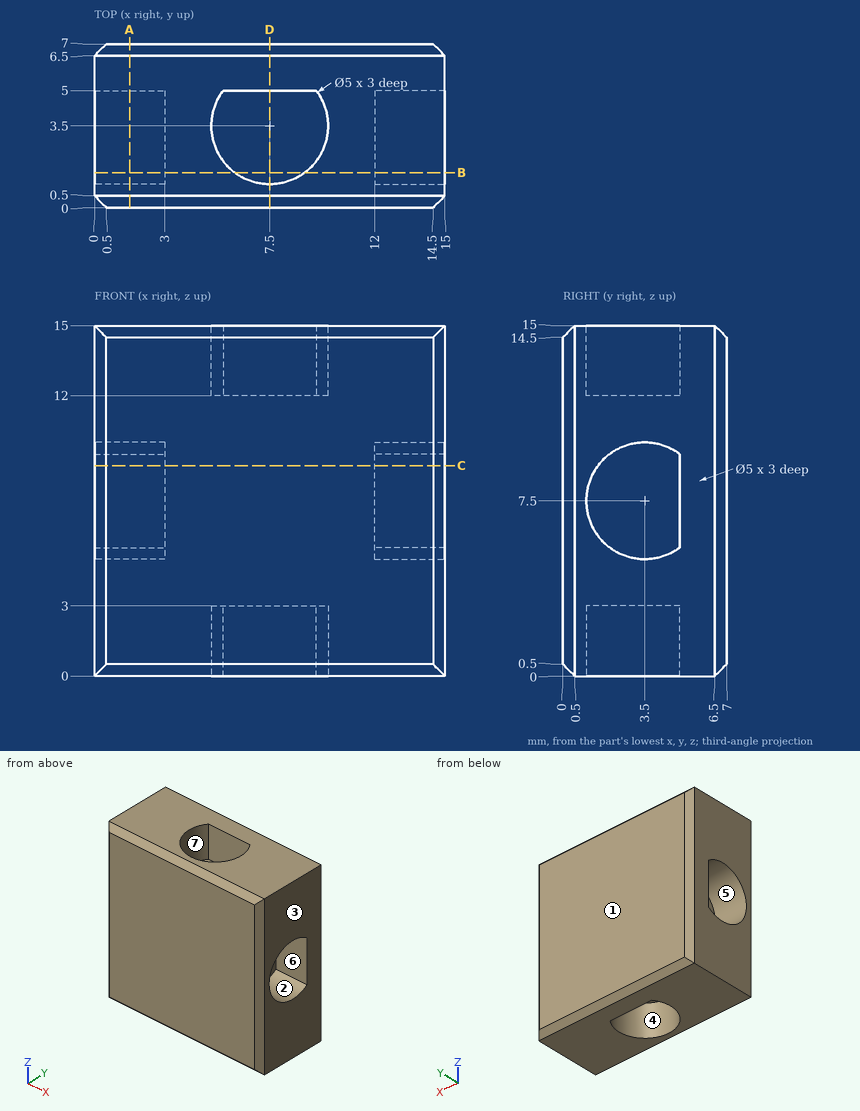
Drawing for the job (mm, zero at the part's lowest x, y, z). A direction names the side the tool comes from. Coordinates: 2 decimals unless noted, no trailing zeros. Order: outer loops, then holes, each group sorted by start corner. A loop starts at its lowest first (then second) coordinate and runs counter-clockwise, first axis right, second up. Notation, with made-up numbers: (43.5, 76) -> (92.5, 76) arc R16 ccw to (92.5, 98) -> close; hole circle Ø8 at (-12, -7). An arc over 180 degrees is marked (long way). Return JSON: item names as keys, results as strings.
Item 1: Slice it at B-B (y = 1.5). Write the cut outline in (x, z), then the cut area to 3 significant figures.
Model answer:
{"outline": "(0, 0) -> (6, 0) -> (6, 3) -> (9, 3) -> (9, 0) -> (15, 0) -> (15, 6) -> (12, 6) -> (12, 9) -> (15, 9) -> (15, 15) -> (9, 15) -> (9, 12) -> (6, 12) -> (6, 15) -> (0, 15) -> (0, 9) -> (3, 9) -> (3, 6) -> (0, 6) -> close", "area": "189 mm²"}
Item 2: Slice it at A-A (x = 1.5). Write the cut outline in (y, z).
Model answer:
{"outline": "(0, 0.5) -> (0.5, 0) -> (6.5, 0) -> (7, 0.5) -> (7, 14.5) -> (6.5, 15) -> (0.5, 15) -> (0, 14.5) -> close; hole (5, 5.5) -> (5, 9.5) arc R2.5 ccw (long way) to start"}
Item 3: Slice it at C-C (z = 9). Write the cut outline in (x, y).
Model answer:
{"outline": "(0, 0.5) -> (0.5, 0) -> (14.5, 0) -> (15, 0.5) -> (15, 1.5) -> (12, 1.5) -> (12, 5) -> (15, 5) -> (15, 6.5) -> (14.5, 7) -> (0.5, 7) -> (0, 6.5) -> (0, 5) -> (3, 5) -> (3, 1.5) -> (0, 1.5) -> close"}
Item 4: Wall check: line 1 along X through (y, z) = (3.5, 0.95); line 2 along Y through (x, z) = (7.5, 1.25). Give the ranges that are in metal, low to high. Write a range as from..to.
Model answer:
{"line 1": "x = 0..5, 10..15", "line 2": "y = 0..1, 5..7"}
Item 5: Pin check, flat tips, straight feed: P1, Ø2, axis at x = 3, z = 13.5, coming from the -Y side; P2, Ø1.2, axis at y = 4, z = 7.5, coming from the -X side; P3, Ø3, axis at x = 8, y = 3, coming from the +Z side. Stop position of each tip, or through.
Model answer:
{"P1": "stops at y = 0", "P2": "stops at x = 3", "P3": "stops at z = 12"}
Item 6: 3-axis set-ups, long thin cutter, end or side, ignore diameter. For the marked faces 4, 5, 6 and 7: which of +Z, -Z, +X, -X, +Y, -Y reach the whole face in a straight line?
Model answer:
{"face 4": "-Z", "face 5": "-X", "face 6": "+X", "face 7": "+Z"}
Item 7: Slice it at D-D (x = 7.5). Write the cut outline in (y, z), then the cut area to 3 significant figures.
Model answer:
{"outline": "(0, 0.5) -> (0.5, 0) -> (1, 0) -> (1, 3) -> (5, 3) -> (5, 0) -> (6.5, 0) -> (7, 0.5) -> (7, 14.5) -> (6.5, 15) -> (5, 15) -> (5, 12) -> (1, 12) -> (1, 15) -> (0.5, 15) -> (0, 14.5) -> close", "area": "80.5 mm²"}
Item 8: Mould opens along Y. For the marked faces 1, 2 and 3 say: pulls with the +Y half, pulls with the -Y half, needs draft (parallel to the pull), parting line crosses it, or undercut.
Model answer:
{"face 1": "pulls with the +Y half", "face 2": "undercut", "face 3": "needs draft"}
